Autodesk Fusion 360 part; units mm, degrees
sketch "Sketch1" plane through (0, 0, 0) normal (0, 0, 1) x (1, 0, 0)
  line L0 (30, -50) -> (-30, -50)
  line L1 (-30, -50) -> (-30, 50)
  line L2 (-30, 50) -> (30, 50)
  line L3 (30, 50) -> (30, -50)
  line L4 (30, -50) -> (-30, 50) construction
  line L5 (-30, -50) -> (30, 50) construction
  dimension "d1" = 60
  dimension "d2" = 100
extrude "Extrude1" add sketch "Sketch1" along normal blind 40
shell "Shell1" thickness 2.5 removed faces 1 at (10, -16.6667, 40)
fillet "Fillet1" radius 3 4 edges at (30, 50, 20) (-30, 50, 20) (30, -50, 20) (-30, -50, 20)
Input: part model. Units: mm. Frame: model coordinates. A direction names the side the tool comes from. Round coordinates to 2 decimals unless told otherwise and drop trailing zeros. Write each loop counter-clockwise with the first axis right and the second up, starting at its lowest first coordinate (ties: lowest second). Pieces come first, ordered by that corner, then holes.
1) Contact query for flat-ended pins moving along their axis: P1, Ø5, axis at x = -7, y = -29.5, coming from the -Z side; P2, Ø1.5, axis at x = -6.5, y = -26.5, coming from the +Z side. Output: stop coordinate, or through.
2) Cut plane A-A (z = 10.5). Return the cut outline in (x, y), then the cut area to 3 significant figures.
3) Draft query along Y for faces 3 (the flat face through (0, 50, 20)), 4 (the flat face through (0, 47.5, 21)), 5 (the cylindrical face through (-29.14, -49.1, 20.28)), 6 (the flat face through (30, 1, 20)). Return one class per face: pulls with the +Y half, pulls with the -Y half, needs draft (parallel to the pull), parting line crosses it, or undercut.
4) Ray query, L1, parallel to Y at x = 14.5, z = 36.5; L2, parallel to X at y = -30, z = 9.5; L3, parallel to Z at x = -24.5, y = 35. Return the intervals inside material, ascending.
5) Reachability of faces 1 (the flat face through (27.5, 1, 21)), 2 (the cylindrical face through (29.14, 49.1, 20.28)) from +Z, -Z, +X, -X, +Y, -Y: full face, straight path, thin tool, end or side. Return the list, or none.
6) Cut plane C-C (x = -6.5). Return the cut outline in (y, z), then the cut area to 4 significant figures.
7) Cut plane B-B (y = -9). Return the cut outline in (x, z), then the cut area to 4 significant figures.
Geometry says:
1. P1: stops at z = 0
1. P2: stops at z = 2.5
2. outline: (-30, -47) arc R3 ccw to (-27, -50) - (27, -50) arc R3 ccw to (30, -47) - (30, 47) arc R3 ccw to (27, 50) - (-27, 50) arc R3 ccw to (-30, 47) - close; hole (-27.5, -47.5) - (27.5, -47.5) - (27.5, 47.5) - (-27.5, 47.5) - close
2. area: 767 mm2
3. face 3: pulls with the +Y half
3. face 4: undercut
3. face 5: pulls with the -Y half
3. face 6: needs draft
4. L1: y = -50 to -47.5, 47.5 to 50
4. L2: x = -30 to -27.5, 27.5 to 30
4. L3: z = 0 to 2.5
5. face 1: +Z
5. face 2: +Z, -Z, +X, +Y
6. outline: (-50, 0) - (50, 0) - (50, 40) - (47.5, 40) - (47.5, 2.5) - (-47.5, 2.5) - (-47.5, 40) - (-50, 40) - close
6. area: 437.5 mm2
7. outline: (-30, 0) - (30, 0) - (30, 40) - (27.5, 40) - (27.5, 2.5) - (-27.5, 2.5) - (-27.5, 40) - (-30, 40) - close
7. area: 337.5 mm2
